Build history of the part. All positions in model axes, mm. Face numbers are marked on the shaded views. A direction names the side the tool comes from. Give positions to 0.01 mm unless a question says otherwise; leave off trailing zeros. Write each loop counter-clockwise with the first axis right and the second up, starting at its lowest first coordinate (ties: lowest second). Pieces come first, ordered by that corner, then holes.
from build123d import *

# Parameters (mm, degrees)
CUT_EXTRUDE2_START = -12.7
SKETCH5_W          = 12.7
SKETCH5_H          = 12.7
CUT_EXTRUDE2_DEPTH = 73.673472495
CIRPATTERN1_COUNT  = 4


with BuildPart() as part:
    # Sketch1 → base_ring (revolve)
    with BuildSketch(Plane.YZ, mode=Mode.PRIVATE) as base_ring_sk:
        Polygon((27.78125, 0), (27.78125, 24.13), (26.51125, 24.13), (26.51125, 33.02), (35.40125, 33.02), (35.40125, 24.13), (30.32125, 0), align=None)
    revolve(base_ring_sk.sketch.rotate(Axis((0, 0, 0), (0, 0, 1)), 90), axis=Axis((0, 0, 0), (0, 0, 1)))

    # Sketch5 → Cut-Extrude2 (cut)
    with BuildSketch(Plane.XY.offset(33.02).offset(CUT_EXTRUDE2_START)):
        with Locations((0, 32.089539168)):
            Rectangle(SKETCH5_W, SKETCH5_H)
    cut_extrude2 = extrude(amount=CUT_EXTRUDE2_DEPTH, mode=Mode.SUBTRACT)

    # Sketch8 → pulley_bolt_hole (revolve, cut)
    with BuildSketch(Plane(origin=(35.40125, 29.747087182, 27.94), x_dir=(0, 0, -1), z_dir=(0, 1, 0))):
        Polygon((0, 0), (0, 39.275163199), (1.9558, 38.1), (1.9558, 22.3012), (3.77063, 22.3012), (3.77063, 0), align=None)
    pulley_bolt_hole = revolve(axis=Axis((41.75125, 29.747087182, 27.94), (-1, 0, 0)), mode=Mode.SUBTRACT)

    # bolthole_mirror: pulley_bolt_hole across plane
    add(pulley_bolt_hole.mirror(Plane(origin=(0, 0, 0), x_dir=(0, 0, 1), z_dir=(1, 0, 0))), mode=Mode.SUBTRACT)

    # CirPattern1: Cut-Extrude2, pulley_bolt_hole ×4 about axis
    cirpattern1_axis = Axis((0, 0, 0), (0, 0, 1))
    add([cut_extrude2.rotate(cirpattern1_axis, i * 360 / CIRPATTERN1_COUNT) for i in range(1, CIRPATTERN1_COUNT)], mode=Mode.SUBTRACT)
    add([pulley_bolt_hole.rotate(cirpattern1_axis, i * 360 / CIRPATTERN1_COUNT) for i in range(1, CIRPATTERN1_COUNT)], mode=Mode.SUBTRACT)

    # CirPattern1 copy 1 sketch → CirPattern1 copy 1 (revolve, cut)
    with BuildSketch(Plane(origin=(-29.747087182, -35.40125, 27.94), x_dir=(0, 0, -1), z_dir=(-1, 0, 0))):
        Polygon((0, 0), (0, -39.275163199), (1.9558, -38.1), (1.9558, -22.3012), (3.77063, -22.3012), (3.77063, 0), align=None)
    revolve(axis=Axis((-29.747087182, -41.75125, 27.94), (0, -1, 0)), mode=Mode.SUBTRACT)

    # CirPattern1 copy 2 sketch → CirPattern1 copy 2 (revolve, cut)
    with BuildSketch(Plane(origin=(35.40125, -29.747087182, 27.94), x_dir=(0, 0, -1), z_dir=(0, -1, 0))):
        Polygon((0, 0), (0, -39.275163199), (1.9558, -38.1), (1.9558, -22.3012), (3.77063, -22.3012), (3.77063, 0), align=None)
    revolve(axis=Axis((41.75125, -29.747087182, 27.94), (1, 0, 0)), mode=Mode.SUBTRACT)

    # CirPattern1 copy 3 sketch → CirPattern1 copy 3 (revolve, cut)
    with BuildSketch(Plane(origin=(29.747087182, 35.40125, 27.94), x_dir=(0, 0, -1), z_dir=(1, 0, 0))):
        Polygon((0, 0), (0, -39.275163199), (1.9558, -38.1), (1.9558, -22.3012), (3.77063, -22.3012), (3.77063, 0), align=None)
    revolve(axis=Axis((29.747087182, 41.75125, 27.94), (0, 1, 0)), mode=Mode.SUBTRACT)


solid = part.part
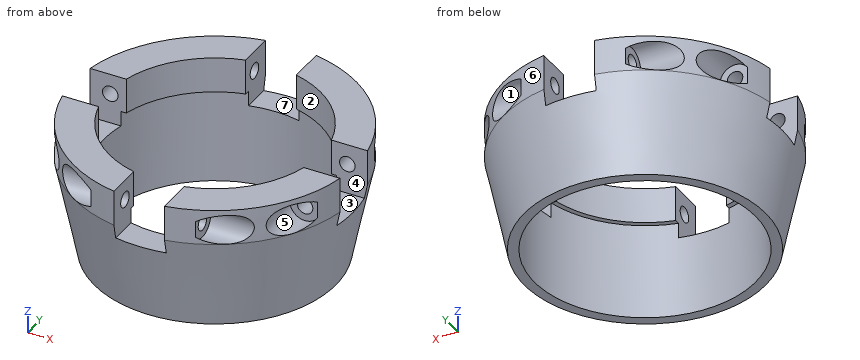
1. 3-axis set-ups, long thin cutter, end or side, ignore diameter. For the marked faces 1, 2 and 3: which of +Z, -Z, +X, -X, +Y, -Y reach the whole face in a straight line?
2. Saw through at A-A on x = 0. Give the cut face in (y, z).
3. Drill centre lines: line 1 along X through (y, z) = (30.5, 31); line 2 along X through (y, z) = (-10, 27.94); line 3 along Y through (x, z) = (17, 27). Where is each one in solid material? Low to high.
4. Drop flat-ended pins along their axis: pin 1 (4.5 mm diameter, centred on y = -29, z = 27.5, fed in from +X); pin 2 (3 mm diameter, centred on x = 12.5, z = 28, fed in from +Y); pin 3 (3.5 mm diameter, centred on x = 29.75, z = 27.94, fed in from +Y); pin 4 (10 mm diameter, centred on x = -32, z = 24, fed in from +Y). Give the stop position or say it passes through.
5. Mould opens along X. For the marked faces 4, 5, 6 and 7 say: pulls with the +X half, pulls with the -X half, needs draft (parallel to the pull), parting line crosses it, or undercut.
6. Saw through at C-C on z = 27.94. Count the separate pieces of the cut face and the enclosed holes in it, plus the area to 3 significant figures.
Outcome:
1. face 1: +X
1. face 2: +Z, -Z
1. face 3: +Z, +X, -X
2. outline: (-34.6, 20.32) - (-30.32, 0) - (-27.78, 0) - (-27.78, 20.32) - close; (27.78, 0) - (30.32, 0) - (34.6, 20.32) - (27.78, 20.32) - close
3. line 1: x = -13.1 to -6.35, 6.35 to 13.1
3. line 2: x = -33.96 to -31.7, -27.79 to -24.55, 24.55 to 27.79, 31.7 to 33.96
3. line 3: y = -26.1 to -20.34, 20.34 to 26.1
4. pin 1: stops at x = 13.1
4. pin 2: stops at y = 33.65
4. pin 3: passes through
4. pin 4: stops at y = 22.89
5. face 4: needs draft
5. face 5: undercut
5. face 6: pulls with the +X half
5. face 7: undercut
6. separate pieces: 12
6. enclosed holes: 0
6. area: 719 mm2
